```python
from build123d import *

# Parameters (mm, degrees)
BOSS_EXTRUDE1_DEPTH = 26
BOSS_EXTRUDE3_DEPTH = 20
BOSS_EXTRUDE4_DEPTH = 4


with BuildPart() as part:
    # Sketch2 → Boss-Extrude1 (new, symmetric)
    with BuildSketch(Plane.XY):
        Polygon((-5, 4), (5, 4), (37.5, 4), (37.5, -4), (-37.5, -4), (-37.5, 4), align=None)
    extrude(amount=BOSS_EXTRUDE1_DEPTH, both=True)

    # Sketch2_4 → Boss-Extrude3 (add, symmetric)
    with BuildSketch(Plane.XY):
        with BuildLine():
            Line((5, 4), (5, 24))
            ThreePointArc((5, 24), (15.811388301, 31.117468017), (20, 43.364916731))
            Line((20, 43.364916731), (12, 43.364916731))
            ThreePointArc((12, 43.364916731), (0, 31.364916731), (-12, 43.364916731))
            Line((-12, 43.364916731), (-20, 43.364916731))
            ThreePointArc((-20, 43.364916731), (-15.811388301, 31.117468017), (-5, 24))
            Line((-5, 24), (-5, 4))
            Line((-5, 4), (5, 4))
        make_face()
    extrude(amount=BOSS_EXTRUDE3_DEPTH, both=True)

    # Sketch2_6 → Boss-Extrude4 (add, symmetric)
    with BuildSketch(Plane.XY):
        with BuildLine():
            ThreePointArc((5, 24), (15.811388301, 31.117468017), (20, 43.364916731))
            Line((20, 43.364916731), (37.5, 4))
            Line((37.5, 4), (5, 4))
            Line((5, 4), (5, 24))
        make_face()
        with BuildLine():
            ThreePointArc((-20, 43.364916731), (-15.811388301, 31.117468017), (-5, 24))
            Line((-5, 24), (-5, 4))
            Line((-5, 4), (-37.5, 4))
            Line((-37.5, 4), (-20, 43.364916731))
        make_face()
    extrude(amount=BOSS_EXTRUDE4_DEPTH, both=True)


solid = part.part
```
Read the model definition and answer for the solid it produces. Units are mm, in the model's axes. A direction names the side the tool comes from. Coordinates: 2 decimals unless noted, no trailing zeros. Write each loop counter-clockwise with the first axis right and the second up, starting at its lowest first coordinate (ties: lowest second). Pieces come first, ordered by that corner, then holes. Notation, with made-up numbers: (9, 26) -> (28, 26) arc R17 ccw to (28, 41) -> close; hole circle Ø8 at (59, 82.5). An arc over 180 degrees is marked (long way). Return JSON: item names as keys, results as strings.
1. A tool of negligible diameter and unlimited length cuts with its end or side. For faces 1 (the face through (1, 4, -22)), 2 (the face through (0, 24, 20)), 3 (the face through (15.698, 30.972, 12.112)), 4 (the face through (15.698, 30.972, -11.888)), 5 (the face through (-17, 20, -4)), from which of +Z, -Z, +X, -X, +Y, -Y can it reach the whole face along a straight path? Write none if from no direction.
Found:
{"face 1": "-Z", "face 2": "+Z, +X, -X, +Y", "face 3": "+Z, +X", "face 4": "-Z, +X", "face 5": "-Z, -X"}
2. A cutting plane is placed at C-C (x = 0). Determine the outline of the cut face in (y, z).
Found:
{"outline": "(-4, -26) -> (4, -26) -> (4, -20) -> (31.36, -20) -> (31.36, 20) -> (4, 20) -> (4, 26) -> (-4, 26) -> close"}
3. Each of these flat-tipped pins is pushed along its axis until it touches: P1, Ø16, axis at x = -18.5, y = 19.5, coming from the -Z side; P2, Ø13, axis at y = 11.5, z = 12, coming from the -X side; P3, Ø6.5, axis at x = 1, z = 19.5, coming from the +Y side. Where does it stop, or does it pass through?
Found:
{"P1": "z = -4", "P2": "x = -5", "P3": "y = 32.14"}
4. Determine the mould class of faces 6 (the face through (28.628, 23.958, -0.056)), 7 (the face through (-5, 14, 12)), 8 (the face through (-37.5, 0, 0)) for opening direction Y: pulls with the +Y half, pulls with the -Y half, needs draft (parallel to the pull), parting line crosses it, or undercut.
Found:
{"face 6": "pulls with the +Y half", "face 7": "undercut", "face 8": "needs draft"}
5. A cutting plane is placed at B-B (z = 2). Determine the outline of the cut face in (x, y).
Found:
{"outline": "(-37.5, -4) -> (37.5, -4) -> (37.5, 4) -> (20, 43.36) -> (12, 43.36) arc R12 cw to (-12, 43.36) -> (-20, 43.36) -> (-37.5, 4) -> close"}
6. A cutting plane is placed at A-A (y = 34.5). Determine the outline of the cut face in (x, z), and give its area (3 significant figures).
Found:
{"outline": "(-23.94, -4) -> (-17.93, -4) -> (-17.93, -20) -> (-8.09, -20) -> (-8.09, 20) -> (-17.93, 20) -> (-17.93, 4) -> (-23.94, 4) -> close; (8.09, -20) -> (17.93, -20) -> (17.93, -4) -> (23.94, -4) -> (23.94, 4) -> (17.93, 4) -> (17.93, 20) -> (8.09, 20) -> close", "area": "883 mm2"}
7. Find the intervals of material crossed by line 1 along X through (y, z) = (14.5, -15); line 2 along Y through (x, z) = (8, 21), in increasing order. Write a range as from..to.
Found:
{"line 1": "-5..5", "line 2": "-4..4"}
8. A cutting plane is placed at D-D (y = 12). Determine the outline of the cut face in (x, z), and give its area (3 significant figures).
Found:
{"outline": "(-33.94, -4) -> (-5, -4) -> (-5, -20) -> (5, -20) -> (5, -4) -> (33.94, -4) -> (33.94, 4) -> (5, 4) -> (5, 20) -> (-5, 20) -> (-5, 4) -> (-33.94, 4) -> close", "area": "863 mm2"}
